from build123d import *

# Parameters (mm, degrees)
TAP_DRILL_FOR_M3X0_5_TAP1_D     = 2.5
TAP_DRILL_FOR_M3X0_5_TAP1_DEPTH = 3
TAP_DRILL_FOR_M3X0_5_TAP1_TIP   = 0.751075774
SKETCH5_W                       = 8
SKETCH5_H                       = 0.5
CUT_EXTRUDE1_DEPTH              = 13.5
CUT_EXTRUDE1_DEPTH_BACK         = 13.5


with BuildPart() as part:
    # Sketch1 → Revolve1 (revolve)
    with BuildSketch(Plane.XY):
        with BuildLine():
            Line((0, 0), (0, 2))
            Line((0, 2), (9, 2))
            ThreePointArc((9, 2), (9.439339828, 3.060660172), (10.5, 3.5))
            Line((10.5, 3.5), (11.5, 3.5))
            Line((11.5, 3.5), (11.5, 12.5))
            Line((11.5, 12.5), (32.5, 12.5))
            Line((32.5, 12.5), (32.5, 10.5))
            ThreePointArc((32.5, 10.5), (33.085786438, 11.914213562), (34.5, 12.5))
            Line((34.5, 12.5), (65.3, 12.5))
            Line((65.3, 12.5), (65.3, 3.5))
            Line((65.3, 3.5), (66.3, 3.5))
            Line((66.3, 3.5), (66.3, 12.5))
            Line((66.3, 12.5), (67.3, 12.5))
            Line((67.3, 12.5), (67.3, 2.5))
            Line((67.3, 2.5), (69.3, 2.5))
            Line((69.3, 2.5), (69.3, 7))
            Line((69.3, 7), (73, 7))
            Line((73, 7), (73, 0))
            Line((73, 0), (0, 0))
        make_face()
    revolve(axis=Axis((0, 0, 0), (1, 0, 0)))

    # Tap Drill for M3x0.5 Tap1
    with Locations(Plane.ZY.offset(-11.5)):
        with Locations((-8.5, 0), (8.5, 0)):
            Hole(TAP_DRILL_FOR_M3X0_5_TAP1_D / 2, depth=TAP_DRILL_FOR_M3X0_5_TAP1_DEPTH)
            with Locations((0, 0, -(TAP_DRILL_FOR_M3X0_5_TAP1_DEPTH + TAP_DRILL_FOR_M3X0_5_TAP1_TIP / 2))):  # 118° drill point
                Cone(0, TAP_DRILL_FOR_M3X0_5_TAP1_D / 2, TAP_DRILL_FOR_M3X0_5_TAP1_TIP, mode=Mode.SUBTRACT)

    # Sketch5 → Cut-Extrude1 (cut, two sides)
    with BuildSketch(Plane.XY) as cut_extrude1_sk:
        with Locations((4, 1.75)):
            Rectangle(SKETCH5_W, SKETCH5_H)
    extrude(amount=CUT_EXTRUDE1_DEPTH, mode=Mode.SUBTRACT)
    extrude(cut_extrude1_sk.sketch, amount=-CUT_EXTRUDE1_DEPTH_BACK, mode=Mode.SUBTRACT)


solid = part.part
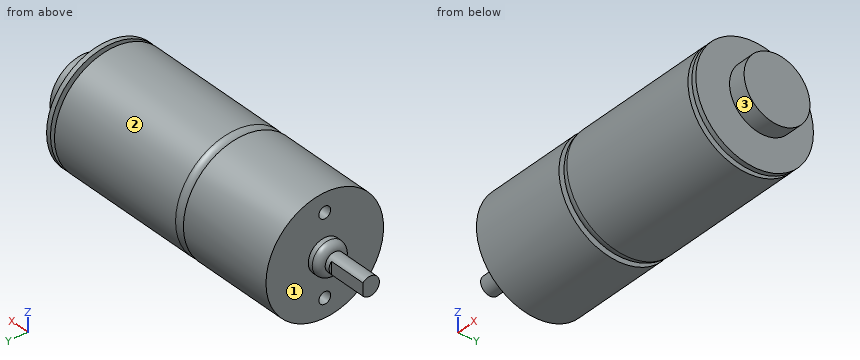
Build history of the part. All positions in model axes, mm. Face numbers are marked on the shaded views. A direction names the side the tool comes from. Give positions to 0.01 mm unless a question says otherwise; leave off trailing zeros. Order: outer loops, then holes, each group sorted by start corner. A loop starts at its lowest first (then second) coordinate and runs counter-clockwise, first axis right, second up. Notation, with made-up numbers: M 3.25,-2.5 L 41.25,-2.5 A15 cw 41.25,8.5 Z; hole C 50,80.5 d8. An arc over 180 degrees is marked long. Put each result on its own line as item: value.
Item 1: Which spindle directions (+Z, -Z, +X, -X, +Y, -Y) get a long thin tool onto all of the face, cutting with end or side? Do the marked faces 1, 2 and 3. Say none if no direction does.
Results are:
face 1: -X
face 2: +X, -X
face 3: +X
Item 2: Cut at A-A on x = 59.5. Write the cut outline in (y, z).
Results are:
outline: C 0,0 d25
Item 3: Wall check: probe 1 along Z at (x, y) = (13.6, 0); probe 2 along X at (y, z) = (-4, 2.5); probe 3 along X at (y, z) = (-6, -7.25). Give the ranges that are in metal, low to high.
Results are:
probe 1: -12.5 to -9.75, -7.25 to 7.25, 9.75 to 12.5
probe 2: 11.5 to 65.3, 66.3 to 67.3, 69.3 to 73
probe 3: 11.5 to 65.3, 66.3 to 67.3
Item 4: Drop flat-ended pins along their axis: pin 1 Ø10 at (x, z) = (55, -4.5) entering from -Y; pin 2 Ø1.3 at (x, z) = (5.5, 0) entering from +Y; pin 3 Ø3 at (x, z) = (63, 2.5) entering from +Y; pin 4 Ø4 at (x, z) = (15.5, 5.5) entering from +Y. Give the stop position or say it passes through.
Results are:
pin 1: y = -12.5
pin 2: y = 1.5
pin 3: y = 12.46
pin 4: y = 12
Item 5: Cut at B-B on y = 5.5. Count the separate pieces of the cut face and the enclosed holes in it, then the cut area to 3 significant figures.
Results are:
separate pieces: 3
enclosed holes: 0
area: 1,260 mm2
